Here's how the part is built. I have some questions about the finished solid (model axes, mm). A direction names the side the tool comes from. Give positions to 0.01 mm unless a question says otherwise; leave off trailing zeros. Write each loop counter-clockwise with the first axis right and the second up, starting at its lowest first coordinate (ties: lowest second). Pieces come first, ordered by that corner, then holes. Notation, with made-up numbers: (8, -20.75) -> (26, -20.75) arc R33 cw to (26, 12.25) -> close; hole circle Ø3 at (-21.5, 45). An arc over 180 degrees is marked (long way). Use CSV: the item, a comma, the result in double quotes. Start each with the question number.
(1) Suppose I cut it at C-C on z = 3.5. Give the number of separate pieces and of enclosed holes in the cut face, plus the area to 3 significant figures.
(2) I need wall thicknesses on L1, parallel to X at y = -0.5, z = 5.5; L2, parallel to Y at x = 16, z = 5.75; L3, parallel to Y at x = 0.5, z = 2.75. Which ranges of each line are inside material? Lowest first, please. Write a range as [from, to].
(3) Suppose I cut it at B-B on x = -16. List the corners of the cut face in (y, z) for me.
(4) For pin 1 Ø3.5 at (x, y) = (-16, 16) entering from -Z; pin 2 Ø3 at (x, z) = (9, 4.5) entering from -Y; pin 3 Ø0.5 at (x, z) = (20, 4) entering from -Y; pin 4 Ø5 at (x, y) = (16, 16) entering from -Z, each with a flat end and sliding along its axis, tell me the tip position at first contact or that it passes through.
(5) Suppose I cut it at D-D on y = 10. List the corners of the cut face in (x, z) for me, plus the area to 3 significant figures.
(6) If we mould it in two halves opening along X, with no side actions, what happens to faces 5 (the flat face through (-11, 16, 7.5)), 6 (the cylindrical face through (-12.84, -14.61, 3.8)), 7 (the cylindrical face through (-19.859, 19.797, 3.802)), 8 (the cylindrical face through (16, -14, 4))? For each: pulls with the +X half, pulls with the -X half, needs draft (parallel to the pull), parting line crosses it, or undercut.
(7) Which directions (+Z, -Z, +X, -X, +Y, -Y) give clear straight access to the entire face, cutting with the end or side of a thin tool? Please do faces 1 (the flat face through (-19.25, 10.49, 3.8)), 2 (the cylindrical face through (-13.641, -19.797, 3.698)), 3 (the flat face through (19.25, 10.49, 3.8)), 4 (the cylindrical face through (12.86, -14.56, 3.8)).
(8) Suppose I cut it at A-A on y = 0. List the corners of the cut face in (x, z) for me.
from build123d import *

# Parameters (mm, degrees)
CROQUIS1_W              = 42
CROQUIS1_H              = 42
SALIENTE_EXTRUIR1_DEPTH = 7.5
CROQUIS2_R              = 19
CORTAR_EXTRUIR1_DEPTH   = 8.5
CROQUIS3_R              = 2
CORTAR_EXTRUIR2_DEPTH   = 8.5
CROQUIS4_W              = 25
CROQUIS4_H              = 33.5
CORTAR_EXTRUIR3_DEPTH   = 8.5
REDONDEO1_R             = 4
REDONDEO2_R             = 5
CORTAR_EXTRUIR4_DEPTH   = 8.5
REDONDEO3_R             = 0.75


with BuildPart() as part:
    # Croquis1 → Saliente-Extruir1 (new body)
    with BuildSketch(Plane.XY):
        Rectangle(CROQUIS1_W, CROQUIS1_H)
    extrude(amount=SALIENTE_EXTRUIR1_DEPTH)

    # Croquis2 → Cortar-Extruir1 (cut, through all)
    with BuildSketch(Plane.XY.offset(7.5)):
        Circle(CROQUIS2_R)
    extrude(amount=-CORTAR_EXTRUIR1_DEPTH, mode=Mode.SUBTRACT)

    # Croquis3 → Cortar-Extruir2 (cut, through all)
    with BuildSketch(Plane.XY.offset(7.5)):
        with Locations((-16, 16)):
            Circle(CROQUIS3_R)
        with Locations((16, 16)):
            Circle(CROQUIS3_R)
        with Locations((16, -16)):
            Circle(CROQUIS3_R)
        with Locations((-16, -16)):
            Circle(CROQUIS3_R)
    extrude(amount=-CORTAR_EXTRUIR2_DEPTH, mode=Mode.SUBTRACT)

    # Croquis4 → Cortar-Extruir3 (cut, through all)
    with BuildSketch(Plane.XY.offset(7.5)):
        with Locations((0, -4.25)):
            Rectangle(CROQUIS4_W, CROQUIS4_H)
    extrude(amount=-CORTAR_EXTRUIR3_DEPTH, mode=Mode.SUBTRACT)

    # Redondeo1
    redondeo1_edges = [part.edges().sort_by_distance(p)[0] for p in [
        (-12.5, -21, 3.75),
        (12.5, -21, 3.75),
        (-21, 21, 3.75),
        (21, 21, 3.75),
        (21, -21, 3.75),
        (-21, -21, 3.75),
    ]]
    fillet(redondeo1_edges, radius=REDONDEO1_R)

    # Redondeo2
    redondeo2_edges = [part.edges().sort_by_distance(p)[0] for p in [
        (12.5, -14.309088021, 3.75),
        (-12.5, -14.309088021, 3.75),
    ]]
    fillet(redondeo2_edges, radius=REDONDEO2_R)

    # Croquis5 → Cortar-Extruir4 (cut, through all)
    with BuildSketch(Plane.XY.offset(7.5)):
        Polygon((-21, 7), (-21, 14), (-19, 14), (-19.5, 7), align=None)
        Polygon((21, 14), (19, 14), (19.5, 7), (21, 7), align=None)
    extrude(amount=-CORTAR_EXTRUIR4_DEPTH, mode=Mode.SUBTRACT)

    # Redondeo3
    redondeo3_edges = [part.edges().sort_by_distance(p)[0] for p in [
        (-19.5, 7, 3.75),
        (-21, 7, 3.75),
        (-21, 14, 3.75),
        (-19, 14, 3.75),
        (21, 14, 3.75),
        (21, 7, 3.75),
        (19.5, 7, 3.75),
        (19, 14, 3.75),
    ]]
    fillet(redondeo3_edges, radius=REDONDEO3_R)


solid = part.part
Geometry says:
1,separate pieces,"1"
1,enclosed holes,"4"
1,area,"447 mm²"
2,L1,"[-21, -18.99], [18.99, 21]"
2,L2,"[-20.97, -18], [-14, -10.25], [10.25, 14], [18, 21]"
2,L3,"[18.99, 21]"
3,outline,"(-20.97, 0) -> (-18, 0) -> (-18, 7.5) -> (-20.97, 7.5) -> close; (-14, 0) -> (-10.25, 0) -> (-10.25, 7.5) -> (-14, 7.5) -> close; (10.25, 0) -> (14, 0) -> (14, 7.5) -> (10.25, 7.5) -> close; (18, 0) -> (21, 0) -> (21, 7.5) -> (18, 7.5) -> close"
4,pin 1,"through"
4,pin 2,"y = 15.84"
4,pin 3,"y = -19.9"
4,pin 4,"z = 0"
5,outline,"(-19.29, 0) -> (-16.16, 0) -> (-16.16, 7.5) -> (-19.29, 7.5) -> close; (16.16, 0) -> (19.29, 0) -> (19.29, 7.5) -> (16.16, 7.5) -> close"
5,area,"47.0 mm²"
6,face 5,"needs draft"
6,face 6,"undercut"
6,face 7,"pulls with the -X half"
6,face 8,"undercut"
7,face 1,"+Z, -Z, -X"
7,face 2,"+Z, -Z, -Y"
7,face 3,"+Z, -Z, +X"
7,face 4,"+Z, -Z"
8,outline,"(-21, 0) -> (-19, 0) -> (-19, 7.5) -> (-21, 7.5) -> close; (19, 0) -> (21, 0) -> (21, 7.5) -> (19, 7.5) -> close"
